from build123d import *

# Parameters (mm, degrees)
SKETCH_1_W          = 15
SKETCH_1_H          = 15
SKETCH_1_W_2        = 12
SKETCH_1_H_2        = 12
EXTRUDE_1_DEPTH     = 267
SKETCH_2_R          = 2.15
CUT_EXTRUDE_1_DEPTH = 268.526166944
SKETCH_3_R          = 2.15
CUT_EXTRUDE_2_DEPTH = 268.526166944


with BuildPart() as part:
    # ｽｹｯﾁ1 → 押し出し-薄板1 (new body)
    with BuildSketch(Plane(origin=(0, 0, 0), x_dir=(0, 0, -1), z_dir=(1, 0, 0))):
        Rectangle(SKETCH_1_W, SKETCH_1_H)
        Rectangle(SKETCH_1_W_2, SKETCH_1_H_2, mode=Mode.SUBTRACT)
    extrude(amount=EXTRUDE_1_DEPTH)

    # ｽｹｯﾁ2 → ｶｯﾄ - 押し出し1 (cut, through all)
    with BuildSketch(Plane(origin=(0, 7.5, 0), x_dir=(1, 0, 0), z_dir=(0, 1, 0))):
        with Locations(Location((262, 0, 0), (0, 0, 270))):
            Circle(SKETCH_2_R)
        with Locations(Location((22, 0, 0), (0, 0, 270))):
            Circle(SKETCH_2_R)
        with Locations(Location((7, 0, 0), (0, 0, 270))):
            Circle(SKETCH_2_R)
        with Locations(Location((237, 0, 0), (0, 0, 270))):
            Circle(SKETCH_2_R)
        with Locations(Location((127, 0, 0), (0, 0, 270))):
            Circle(SKETCH_2_R)
    extrude(amount=-CUT_EXTRUDE_1_DEPTH, mode=Mode.SUBTRACT)

    # ｽｹｯﾁ3 → ｶｯﾄ - 押し出し2 (cut, through all)
    with BuildSketch(Plane.XY.offset(7.5)):
        with Locations((247, 0)):
            Circle(SKETCH_3_R)
    extrude(amount=-CUT_EXTRUDE_2_DEPTH, mode=Mode.SUBTRACT)


solid = part.part
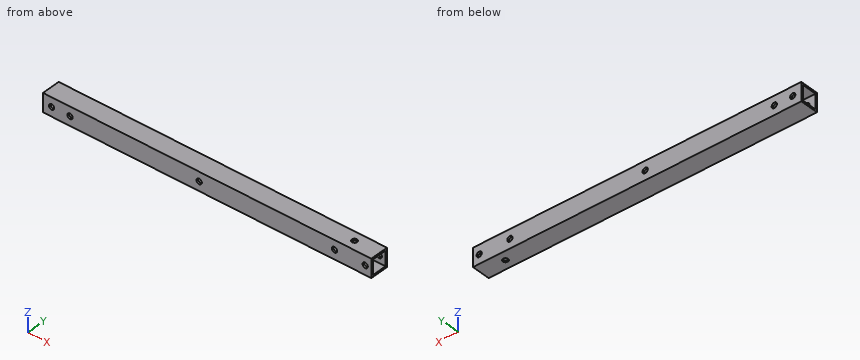
Here's how the part is built. I have some questions about the finished solid (model axes, mm). Coordinates: 2 decimals unless noted, no trailing zeros. Write each loop counter-clockwise with the first axis right and the second up, starting at its lowest first coordinate (ties: lowest second). Pieces come first, ordered by that corner, then holes.
Item 1: I want a section at C-C on x = 80.5. Write out the boundary of the cut face in (y, z), and give its area (3 significant figures).
Item 2: Will this pin go through, and if not, where does the flat tip stop? pin 1 (4 mm diameter, centred on x = 237, z = 0, fed in from +Y).
Item 3: If I drill on line 1 (X direction, y = 6.75, z = 0); line 2 (Y direction, x = 69, z = -2.5), over which ranges is the centre line in solid material (lowest first)?
Item 4: I want a section at B-B on x = 7. Write out the boundary of the cut face in (y, z).
Item 5: I want a section at A-A on y = 0. Write out the boundary of the cut face in (x, z), and give its area (3 significant figures).
Findings below:
1. outline: (-7.5, -7.5) - (7.5, -7.5) - (7.5, 7.5) - (-7.5, 7.5) - close; hole (-6, -6) - (6, -6) - (6, 6) - (-6, 6) - close
1. area: 81.0 mm2
2. pin 1: passes through
3. line 1: x = 0 to 4.85, 9.15 to 19.85, 24.15 to 124.85, 129.15 to 234.85, 239.15 to 259.85, 264.15 to 267
3. line 2: y = -7.5 to -6, 6 to 7.5
4. outline: (-7.5, -7.5) - (7.5, -7.5) - (7.5, -2.15) - (6, -2.15) - (6, -6) - (-6, -6) - (-6, -2.15) - (-7.5, -2.15) - close; (-7.5, 2.15) - (-6, 2.15) - (-6, 6) - (6, 6) - (6, 2.15) - (7.5, 2.15) - (7.5, 7.5) - (-7.5, 7.5) - close
5. outline: (0, -7.5) - (244.85, -7.5) - (244.85, -6) - (0, -6) - close; (0, 6) - (244.85, 6) - (244.85, 7.5) - (0, 7.5) - close; (249.15, -7.5) - (267, -7.5) - (267, -6) - (249.15, -6) - close; (249.15, 6) - (267, 6) - (267, 7.5) - (249.15, 7.5) - close
5. area: 788 mm2
